Here's how the part is built. I have some questions about the finished solid (model axes, mm). Face numbers are marked on the shaded views. A direction names the side the tool comes from. Coordinates: 2 decimals unless noted, no trailing zeros. Write each loop counter-clockwise with the first axis right and the second up, starting at its lowest first coordinate (ties: lowest second). Pieces come first, ordered by that corner, then holes. Notation, with made-up numbers: (-21, -27.75) -> (-3, -27.75) arc R15 ccw to (-3, -2.75) -> close; hole circle Ø8 at (39, -13). An arc over 180 degrees is marked (long way). Use a Markdown table: item, result. Add a question column.
Item 1: Imagine slicing it at B-B, the plane x = -109. Write out the boundary of the cut face in (y, z) (3 decimals).
Item 2: Will these pins go through, and if not, where does the flat tip stop? pin 1 Ø10 at (x, z) = (-80.5, -36.5) entering from +Y; pin 2 Ø1.5 at (y, z) = (25.5, -47.5) entering from +X; pin 3 Ø1 at (x, z) = (7, -60) entering from +Y.
Item 3: On a 3-axis mill with a long thin cutter (end or side, diameter ignored), from which of +Z, -Z, +X, -X, +Y, -Y can I reach the whole of each face in a straight line? I mean the marked faces 1, 2 and 3. Say none if no direction works.
Item 4: Imagine slicing it at D-D, the plane x = -67.5. Write out the boundary of the cut face in (y, z), and give its area (3 significant figures).
Item 5: If I drill on line 1 along Y through (x, z) = (-98, -19); line 2 along Z through (x, y) = (-116, 69); line 3 along X through (y, z) = (51, -38), over which ranges is the centre line in solid material (lowest first)? Write a range as from..to.
Item 6: Imagine slicing it at A-A, the plane z = -19.05. Write out the boundary of the cut face in (x, y) (3 decimals).
Item 7: Imagine slicing it at C-C, the plane y = 69.85. Write out the boundary of the cut face in (x, z) (3 decimals).
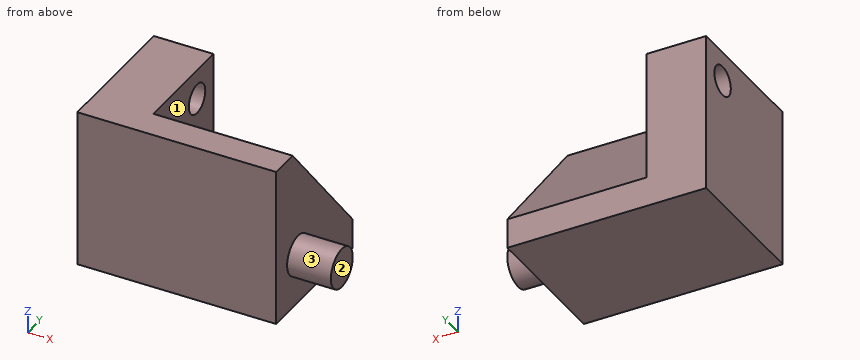
```python
from build123d import *

# Parameters (mm, degrees)
SKETCH1_W           = 88.9
SKETCH1_H           = 82.55
BOSS_EXTRUDE1_DEPTH = 19.05
BOSS_EXTRUDE2_DEPTH = 88.9
BOSS_EXTRUDE3_DEPTH = 88.9
SKETCH5_R           = 9.525
CUT_EXTRUDE1_DEPTH  = 88.9
SKETCH6_R           = 12.7
BOSS_EXTRUDE4_DEPTH = 27.94


with BuildPart() as part:
    # Sketch1 → Boss-Extrude1 (new body)
    with BuildSketch(Plane(origin=(0, 0, 0), x_dir=(1, 0, 0), z_dir=(0, 1, 0))):
        with Locations((-44.45, 41.275)):
            Rectangle(SKETCH1_W, SKETCH1_H)
    extrude(amount=BOSS_EXTRUDE1_DEPTH)

    # Sketch1_3 → Boss-Extrude2 (add)
    with BuildSketch(Plane(origin=(0, 0, 0), x_dir=(1, 0, 0), z_dir=(0, 1, 0))):
        Polygon((-88.9, 82.55), (0, 82.55), (0, 101.6), (-127, 101.6), (-127, 82.55), (-127, 0), (-88.9, 0), align=None)
    extrude(amount=BOSS_EXTRUDE2_DEPTH)

    # Sketch2 → Boss-Extrude3 (add)
    with BuildSketch(Plane(origin=(-88.9, 0, 0), x_dir=(0, 0, -1), z_dir=(1, 0, 0))):
        Polygon((0, 19.05), (82.55, 88.9), (82.55, 19.05), align=None)
    extrude(amount=BOSS_EXTRUDE3_DEPTH)

    # Sketch5 → Cut-Extrude1 (cut)
    with BuildSketch(Plane(origin=(-88.9, 0, 0), x_dir=(0, 0, -1), z_dir=(1, 0, 0))):
        with Locations((19.05, 69.85)):
            Circle(SKETCH5_R)
    extrude(amount=-CUT_EXTRUDE1_DEPTH, mode=Mode.SUBTRACT)

    # Sketch6 → Boss-Extrude4 (add)
    with BuildSketch(Plane(origin=(0, 0, 0), x_dir=(0, 0, -1), z_dir=(1, 0, 0))):
        with Locations(Location((69.85, 25.4, 0), (0, 0, 180))):
            Circle(SKETCH6_R)
    extrude(amount=BOSS_EXTRUDE4_DEPTH)


solid = part.part
```
Ans:
| question | item | result |
|---|---|---|
| 1 | outline | (0, -101.6) -> (88.9, -101.6) -> (88.9, 0) -> (0, 0) -> close; hole circle Ø19.05 at (69.85, -19.05) |
| 2 | pin 1 | stops at y = 54.17 |
| 2 | pin 2 | stops at x = 0 |
| 2 | pin 3 | stops at y = 33.99 |
| 3 | face 1 | +Z, +X, +Y |
| 3 | face 2 | +Z, -Z, +X, +Y, -Y |
| 3 | face 3 | +X |
| 4 | outline | (0, -101.6) -> (88.9, -101.6) -> (88.9, -82.55) -> (19.05, 0) -> (0, 0) -> close |
| 4 | area | 6,150 mm^2 |
| 5 | line 1 | y = 0..60.33, 79.37..88.9 |
| 5 | line 2 | z = -101.6..-28.54, -9.56..0 |
| 5 | line 3 | x = -127..0 |
| 6 | outline | (-127, 0) -> (0, 0) -> (0, 35.169) -> (-88.9, 35.169) -> (-88.9, 60.325) -> (-127, 60.325) -> close; (-127, 79.375) -> (-88.9, 79.375) -> (-88.9, 88.9) -> (-127, 88.9) -> close |
| 7 | outline | (-127, -101.6) -> (0, -101.6) -> (0, -60.036) -> (-88.9, -60.036) -> (-88.9, -28.575) -> (-127, -28.575) -> close; (-127, -9.525) -> (-88.9, -9.525) -> (-88.9, 0) -> (-127, 0) -> close |
